```python
from build123d import *

# Parameters (mm, degrees)
BOSS_EXTRUDE1_DEPTH      = 3.75
BOSS_EXTRUDE1_DEPTH_BACK = 3.75
SKETCH1_R                = 11.92
SKETCH1_R_2              = 9.92
FILLET1_R                = 0.7
FILLET3_R                = 0.7
CUT_REVOLVE2_START       = -3.05
CUT_REVOLVE2_DEPTH       = 6.1


# Read off the part's stored shape, not the designer's step: Cut-Revolve2
with BuildPart() as part:
    # Sketch1 → Boss-Extrude1 (new, two sides: drawn at the far end of the back side and taken through both)
    with BuildSketch(Plane(origin=(0, 0, 0), x_dir=(1, 0, 0), z_dir=(0, 1, 0)).offset(-BOSS_EXTRUDE1_DEPTH_BACK)):
        with Locations(Location((0, 0, 0), (0, 0, 270))):
            Circle(SKETCH1_R)
        with Locations(Location((0, 0, 0), (0, 0, 270))):
            Circle(SKETCH1_R_2, mode=Mode.SUBTRACT)
    extrude(amount=BOSS_EXTRUDE1_DEPTH + BOSS_EXTRUDE1_DEPTH_BACK)

    # Fillet1
    fillet1_edges = [part.edges().sort_by_distance(p)[0] for p in [
        (0, -3.75, -11.92),
        (0, 3.75, -11.92),
    ]]
    fillet(fillet1_edges, radius=FILLET1_R)

    # Sketch3 → Cut-Revolve1 (revolve, cut)
    with BuildSketch(Plane(origin=(0, 0, 0), x_dir=(0, 0, -1), z_dir=(1, 0, 0)), mode=Mode.PRIVATE) as cut_revolve1_sk:
        with BuildLine():
            Line((-9.92, 3.75), (-9.92, 0.005))
            ThreePointArc((-9.92, 0.005), (-10.051616425, 1.893305551), (-10.42, 3.75))
            Line((-10.42, 3.75), (-9.92, 3.75))
        make_face()
        with BuildLine():
            Line((-9.92, -3.75), (-10.42, -3.75))
            ThreePointArc((-10.42, -3.75), (-10.051616425, -1.893305551), (-9.92, -0.005))
            Line((-9.92, -0.005), (-9.92, -3.75))
        make_face()
    revolve(cut_revolve1_sk.sketch.rotate(Axis((0, 0, 0), (0, 1, 0)), 180), axis=Axis((0, 0, 0), (0, 1, 0)), mode=Mode.SUBTRACT)

    # Fillet3
    fillet3_edges = [part.edges().sort_by_distance(p)[0] for p in [
        (0, 3.75, 10.42),
        (0, -3.75, 10.42),
    ]]
    fillet(fillet3_edges, radius=FILLET3_R)

    # Cut-Revolve2 outline → Cut-Revolve2 (cut)
    with BuildSketch(Plane(origin=(0, 0, 0), x_dir=(1, 0, 0), z_dir=(0, 1, 0)).offset(CUT_REVOLVE2_START)):
        with BuildLine():
            ThreePointArc((-8.262613825, 6.671852275), (0, 10.62), (8.262613825, 6.671852275))
            Line((8.262613825, 6.671852275), (9.274044896, 7.488557356))
            ThreePointArc((9.274044896, 7.488557356), (0, 11.92), (-9.274044896, 7.488557356))
            Line((-9.274044896, 7.488557356), (-8.262613825, 6.671852275))
        make_face()
    cut_revolve2 = extrude(amount=CUT_REVOLVE2_DEPTH, mode=Mode.SUBTRACT)

    # Mirror3: Cut-Revolve2 across plane
    add(cut_revolve2.mirror(Plane.XY), mode=Mode.SUBTRACT)


solid = part.part
```
Design review of the part built by this model. Coordinates are the model's own, in mm. A direction names the side the tool comes from. Coordinates: 2 decimals unless noted, no trailing zeros. Order: outer loops, then holes, each group sorted by start corner. A loop starts at its lowest first (then second) coordinate and runs counter-clockwise, first axis right, second up. Notation, with made-up numbers: M 72.5,10.25 L 103.5,10.25 A36 cw 103.5,44.25 Z; hole C 55,5 d3. An arc over 180 degrees is marked long. Answer as a JSON object with one key per item and string values. Group by question number.
1) Add section B-B, the plane y = -1. Write out the cut boundary in (x, z).
2) For pin 1 (2.5 mm diameter, centred on x = 0.5, z = -9.5, fed in from -Y); pin 2 (4 mm diameter, centred on x = -0.5, y = -1, fed in from +Z), all flat-tipped, find the tip position at first contact; note any pin that passes through.
3) Tool access review of faces 1 (the flat face through (0, -3.05, 11)), 2 (the flat face through (8.761, -0.043, -7.074)): name each direction out of +Z, -Z, +X, -X, +Y, -Y from which nothing blocks a thin tool from reaching the whole face with its end or side.
4) Add section A-A, the plane y = 0.5. Write out the cut boundary in (x, z).
5) Mouldability with a two-part tool opening along X and no side actions: class faces 3 (the flat face through (-8.78, -0.04, -7.09)), 4 (the flat face through (-8.78, -0.04, 7.09)), 5 (the cylindrical face through (11.92, -0.04, 0.11)), 6 (the cylindrical face through (-11.92, -0.04, -0.11)) as pulls with the +X half, pulls with the -X half, needs draft (parallel to the pull), parting line crosses it, or undercut.
6) Wall thickness on L1, parallel to X at y = 0.05, z = 0; L2, parallel to X at y = 2.5, z = -6.75; L3, parallel to Z at x = 3.5, y = 0.75: over which ranges is each line inside the solid? List them lowest first.
Computed values:
{
 "1": {"outline": "M -9.27,-7.49 L -8.26,-6.67 A10.62 ccw 8.26,-6.67 L 9.27,-7.49 A11.92 ccw 9.27,7.49 L 8.26,6.67 A10.62 ccw -8.26,6.67 L -9.27,7.49 A11.92 ccw Z; hole C 0,0 d19.92"},
 "2": {"pin 1": "stops at y = -3.72", "pin 2": "stops at z = 10.62"},
 "3": {"face 1": "+Z", "face 2": "-Z"},
 "4": {"outline": "M -9.27,-7.49 L -8.26,-6.67 A10.62 ccw 8.26,-6.67 L 9.27,-7.49 A11.92 ccw 9.27,7.49 L 8.26,6.67 A10.62 ccw -8.26,6.67 L -9.27,7.49 A11.92 ccw Z; hole C 0,0 d19.86"},
 "5": {"face 3": "undercut", "face 4": "undercut", "face 5": "pulls with the +X half", "face 6": "pulls with the -X half"},
 "6": {"L1": "x = -11.92 to -9.92, 9.92 to 11.92", "L2": "x = -9.82 to -8.36, -8.2 to -7.57, 7.57 to 8.2, 8.36 to 9.82", "L3": "z = -10.03 to -9.31, 9.31 to 10.03"}
}
